Verification items for the finished model (mm, model axes). Face numbers are marked on the shaded views. A direction names the side the tool comes from. Give positions to 0.01 mm unless a question says otherwise; leave off trailing zeros. Loops run counter-clockwise (first coordinate to the right, second up) from the corner with the lowest first, then second, coordinate; pieces in that order, holes last. Notation, with made-up numbers: (51.25, 43) -> (76.25, 43) arc R26 ccw to (76.25, 69) -> close; hole circle Ø4 at (37.5, 67). An arc over 180 degrees is marked (long way). Answer in a Markdown table with one row per item. Add a question column.
Q1. Set-up check for the marked faces 4, 5 and 6: record each of +Z, -Z, +X, -X, +Y, -Y from which the full face is reachable in a straight line by a thin tool's end or side.
Q2. Release check for a two-part mould opening along Y. For the marked faces 1, 2 and 3 record: pulls with the +Y half, pulls with the -Y half, needs draft (parallel to the pull), parting line crosses it, or undercut.
Q3. Section check A-A on z = 20. Enter the section's corners in (x, y).
Q4. Section check D-D on y = 4.5. Enter the section's corners in (x, z), and give its area (3 significant figures).
Q5. Section check C-C on y = -7.5. Enter the section's corners in (x, z), and give its area (3 significant figures).
Q6. Material ranges on probe 1 along Z at (x, y) = (4.75, 7.5); probe 2 along X at (y, z) = (-13, 15); probe 3 along Z at (x, y) = (11.25, -11), recorded low to high.
Q7. Gauge pin test, flat ends, axial feed: P1, Ø4, axis at y = 5.5, z = 14.5, coming from the +X side; P2, Ø1, axis at x = 12, y = 6, coming from the +Z side; P3, Ø6, axis at x = 10.5, z = -15, coming from the -Y side. Record the tip position at first contact, or that the pin passes through.
Q8. Section check B-B on x = 4.75. Enter the section's corners in (y, z), and give its area (3 significant figures).
```python
from build123d import *

# Parameters (mm, degrees)
F0_W     = 30
F0_H     = 50
F1_DEPTH = 10
F2_W     = 30
F2_H     = 20
F3_DEPTH = 10
F4_R     = 37
F5_DEPTH = 25.001
F6_DEPTH = 25.001
F7_R     = 1.5
F8_DEPTH = 10.001


with BuildPart() as f1:
    # F0 (on Right) → F1 (new body)
    with BuildSketch(Plane.YZ):
        Rectangle(F0_W, F0_H)
    extrude(amount=F1_DEPTH)

    # F2 (on face) → F3 (join)
    with BuildSketch(Plane.YZ.offset(10)):
        Rectangle(F2_W, F2_H)
    extrude(amount=F3_DEPTH)

    # F4 (on Top) → F5 (cut, through all)
    with BuildSketch(Plane.XY):
        with Locations((47.141809, 0)):
            Circle(F4_R)
    extrude(amount=-F5_DEPTH, mode=Mode.SUBTRACT)

    # F4 (on Top) → F6 (cut, through all)
    with BuildSketch(Plane.XY):
        with Locations((47.141809, 0)):
            Circle(F4_R)
    extrude(amount=F6_DEPTH, mode=Mode.SUBTRACT)

    # F7 (on face) → F8 (cut, through all)
    with BuildSketch(Plane.YZ.offset(10)):
        with Locations((-7.5, 20)):
            Circle(F7_R)
        with Locations((7.5, 20)):
            Circle(F7_R)
        with Locations((-7.5, -20)):
            Circle(F7_R)
        with Locations((7.5, -20)):
            Circle(F7_R)
    extrude(amount=-F8_DEPTH, mode=Mode.SUBTRACT)


solid = f1.part
```
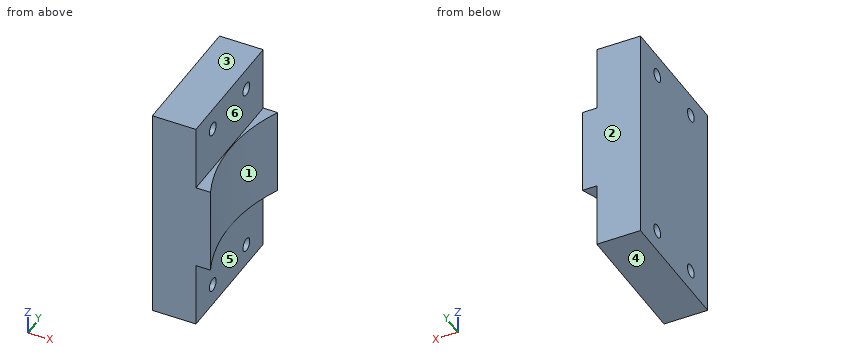
Taken from the geometry:
| question | item | result |
|---|---|---|
| 1 | face 4 | -Z, +X, -X, +Y, -Y |
| 1 | face 5 | -Z, +X, +Y, -Y |
| 1 | face 6 | +Z, +X, +Y, -Y |
| 2 | face 1 | undercut |
| 2 | face 2 | pulls with the +Y half |
| 2 | face 3 | needs draft |
| 3 | outline | (0, -15) -> (10, -15) -> (10, -9) -> (0, -9) -> close; (0, -6) -> (10, -6) -> (10, 6) -> (0, 6) -> close; (0, 9) -> (10, 9) -> (10, 15) -> (0, 15) -> close |
| 4 | outline | (0, -25) -> (10, -25) -> (10, -10) -> (10.42, -10) -> (10.42, 10) -> (10, 10) -> (10, 25) -> (0, 25) -> close |
| 4 | area | 508 mm² |
| 5 | outline | (0, -25) -> (10, -25) -> (10, -21.5) -> (0, -21.5) -> close; (0, -18.5) -> (10, -18.5) -> (10, -10) -> (10.91, -10) -> (10.91, 10) -> (10, 10) -> (10, 18.5) -> (0, 18.5) -> close; (0, 21.5) -> (10, 21.5) -> (10, 25) -> (0, 25) -> close |
| 5 | area | 458 mm² |
| 6 | probe 1 | z = -25 to -21.5, -18.5 to 18.5, 21.5 to 25 |
| 6 | probe 2 | x = 0 to 10 |
| 6 | probe 3 | z = -10 to 10 |
| 7 | P1 | stops at x = 10 |
| 7 | P2 | passes through |
| 7 | P3 | stops at y = -15 |
| 8 | outline | (-15, -25) -> (15, -25) -> (15, 25) -> (-15, 25) -> close; hole circle Ø3 at (-7.5, -20); hole circle Ø3 at (-7.5, 20); hole circle Ø3 at (7.5, -20); hole circle Ø3 at (7.5, 20) |
| 8 | area | 1,470 mm² |
